Check sheet for the modelled part. Datum: model origin and axes. Units: mm. A direction names the side the tool comes from. Give positions to 0.01 mm unless a question says otherwise; leave off trailing zeros. Loops run counter-clockwise (first coordinate to the right, second up) from the corner with the lowest first, then second, coordinate; pieces in that order, holes last. Notation, with made-up numbers: M 2.25,27.5 L 43.25,27.5 A35 ccw 43.25,61.5 Z; hole C 39.5,-6.75 d3. An arc over 180 degrees is marked long. One line per question, with ' | ' between items. Start each with the question number.
Autodesk Inventor part; units mm, degrees
ref_plane "YZ Plane" through (0, 0, 0) normal (1, 0, 0) x (0, 1, 0)
ref_plane "XZ Plane" through (0, 0, 0) normal (0, 1, 0) x (-1, 0, 0)
ref_plane "XY Plane" through (0, 0, 0) normal (0, 0, 1) x (1, 0, 0)
sketch "Boceto2" plane through (0, 0, 0) normal (0, 1, 0) x (-1, 0, 0)
  line L0 (7.5, 100) -> (-7.5, 100)
  line L1 (-7.5, 100) -> (-7.5, -100)
  line L2 (-7.5, -100) -> (7.5, -100)
  line L3 (7.5, -100) -> (7.5, 100)
  line L4 (7.5, 100) -> (-7.5, -100) construction
  line L5 (-7.5, 100) -> (7.5, -100) construction
  point P0 (0, 0)
  dimension "d7" = 15
  dimension "d8" = 200
extrude "Extrusión1" add sketch "Boceto2" along normal blind 10
sketch "Boceto3" plane through (0, 10, 0) normal (0, 1, 0) x (1, 0, 0)
  circle A0 centre (3.25, 58.25) radius 1.75
  line L0 (5, 50) -> (-5, 50)
  line L1 (-5, 50) -> (-5, 60)
  line L2 (-5, 60) -> (5, 60)
  line L3 (5, 60) -> (5, 50)
  line L4 (5, 50) -> (-5, 60) construction
  line L5 (-5, 50) -> (5, 60) construction
  circle A1 centre (-3.25, 51.75) radius 1.75
  line L6 (7.5, 100) -> (-7.5, 100)
  line L7 (-7.5, 0) -> (3.408, 0)
  line L8 (5, -60) -> (5, -50)
  line L9 (-5, -60) -> (5, -60)
  line L10 (5, -50) -> (-5, -50)
  line L11 (-5, -50) -> (-5, -60)
  line L12 (-5, -50) -> (5, -60) construction
  circle A2 centre (-3.25, -51.75) radius 1.75
  line L13 (5, -50) -> (-5, -60) construction
  circle A3 centre (3.25, -58.25) radius 1.75
  line L14 (-7.5, -100) -> (7.5, -100)
  point P0 (0, 0)
  point P1 (-5, 55)
  point P2 (0, 100)
  point P3 (-5, -55)
  dimension "d11" = 3.5
  dimension "d12" = 1.75
  dimension "d13" = 1.75
  dimension "d14" = 1.75
  dimension "d15" = 1.75
  dimension "d16" = 10
  dimension "d17" = 10
  dimension "d19" = 40
  dimension "d81" = 40
hole "Agujero1" at (3.25, 10, 58.25) at (-3.25, 10, 51.75) at (3.25, 10, -58.25) at (-3.25, 10, -51.75) direction (0, -1, 0) diameter 3.5 end through all
sketch "Boceto4" plane through (0, 10, 0) normal (0, 1, 0) x (1, 0, 0)
  line L0 (-7.5, 100) -> (-7.5, -100)
  line L1 (-7.5, -100) -> (7.5, -100)
  line L2 (7.5, -100) -> (7.5, -80)
  line L3 (7.5, -80) -> (-7.5, -80)
  line L4 (-7.5, -80) -> (-7.5, -100)
  line L5 (-7.5, 0) -> (1.0116, 0)
  line L6 (-7.5, -100) -> (-7.5, 100)
  line L7 (-7.5, 100) -> (7.5, 100)
  line L8 (7.5, 100) -> (7.5, 80)
  line L9 (7.5, 80) -> (-7.5, 80)
  line L10 (-7.5, 80) -> (-7.5, 100)
  point P0 (0, 0)
  point P1 (-7.5, -80)
  point P2 (-7.5, 80)
  dimension "d27" = 15
  dimension "d28" = 20
extrude "Extrusión2" add sketch "Boceto4" along normal blind 80
sketch "Boceto5" plane through (0, 90, 0) normal (0, 1, 0) x (1, 0, 0)
  line L0 (-7.5, -100) -> (7.5, -100)
  line L1 (-7.5, -100) -> (49.5, -100)
  line L2 (49.5, -100) -> (49.5, 100)
  line L3 (49.5, 100) -> (-7.5, 100)
  line L4 (-7.5, 100) -> (-7.5, -100)
  line L5 (49.5, -100) -> (-150.5, -100)
  line L6 (-150.5, -100) -> (-150.5, 100)
  line L7 (-150.5, 100) -> (49.5, 100)
  line L8 (49.5, 100) -> (49.5, -100)
  point P0 (0, 0)
  point P1 (-7.5, 100)
  dimension "d31" = 57
  dimension "d32" = 200
  dimension "d75" = 200
extrude "Extrusión3" add sketch "Boceto5" along normal blind 110
sketch "Boceto6" plane through (0, 200, 0) normal (0, 1, 0) x (1, 0, 0)
  line L0 (49.5, 100) -> (7.5, 100)
  line L1 (49.5, 100) -> (29.5, 100)
  line L2 (29.5, 100) -> (29.5, 80)
  line L3 (7.5, -100) -> (49.5, -100)
  line L4 (28.5, -100) -> (28.5, -80)
  line L5 (-150.5, 100) -> (-150.5, -100)
  line L6 (29.5, 80) -> (-150.5, 80)
  line L7 (-150.5, 80) -> (-150.5, -80)
  line L8 (-150.5, -80) -> (29.5, -80)
  line L9 (29.5, -80) -> (29.5, 80)
  line L10 (-150.5, -100) -> (49.5, -100)
  point P0 (7.5, 80)
  point P1 (-50.5, -100)
  dimension "d36" = 20
  dimension "d37" = 20
  dimension "d38" = 20
  dimension "d77" = 20
extrude "Extrusión4" cut sketch "Boceto6" against normal blind 90 contours L8 L5 L6 L9
sketch "Boceto7" plane through (-150.5, 90, -100) normal (-1, 0, 0) x (0, 0, 1)
  line L0 (0, 110) -> (20, 110)
  line L1 (20, 110) -> (10, 110)
  line L2 (10, 110) -> (10, 20)
  line L3 (10, 20) -> (20, 20)
  line L4 (20, 20) -> (20, 110)
  line L5 (180, 110) -> (180, 20)
  line L6 (180, 110) -> (190, 110)
  line L7 (190, 110) -> (190, 20)
  line L8 (190, 20) -> (180, 20)
  line L9 (180, 20) -> (180, 110)
  line L10 (200, 0) -> (200, 110)
  line L11 (0, 0) -> (0, 110)
  line L12 (0, 110) -> (10, 110)
  line L13 (10, 110) -> (10, 20)
  line L14 (10, 20) -> (0, 20)
  line L15 (0, 20) -> (0, 110)
  line L16 (200, 110) -> (0, 110)
  line L17 (200, 110) -> (190, 110)
  line L18 (190, 110) -> (190, 20)
  line L19 (190, 20) -> (200, 20)
  line L20 (200, 20) -> (200, 110)
  point P0 (100, -90)
  dimension "d63" = 10
  dimension "d65" = 10
  dimension "d76" = 10
extrude "Extrusión5" cut sketch "Boceto7" against normal blind 30 contours L6 L7 L8 L5 | L0 L4 L3 L2
sketch "Boceto8" plane through (-7.5, 0, 100) normal (0, 0, 1) x (1, 0, 0)
  line L0 (-113, 110) -> (-113, 200)
  line L1 (-113, 200) -> (-113, 110)
  circle A0 centre (-124.75, 183.25) radius 1.75
  line L2 (-123, 175) -> (-133, 175)
  line L3 (-133, 175) -> (-133, 185)
  line L4 (-133, 185) -> (-123, 185)
  line L5 (-123, 185) -> (-123, 175)
  line L6 (-123, 175) -> (-133, 185) construction
  line L7 (-133, 175) -> (-123, 185) construction
  circle A1 centre (-131.25, 176.75) radius 1.75
  line L8 (-143, 200) -> (57, 200)
  line L9 (-143, 90) -> (-143, 200)
  line L10 (-113, 155) -> (-128, 155)
  line L11 (-123, 125) -> (-123, 135)
  line L12 (-133, 125) -> (-123, 125)
  line L13 (-123, 135) -> (-133, 125) construction
  line L14 (-123, 135) -> (-133, 135)
  line L15 (-133, 135) -> (-123, 125) construction
  circle A2 centre (-131.25, 133.25) radius 1.75
  line L16 (-133, 135) -> (-133, 125)
  circle A3 centre (-124.75, 126.75) radius 1.75
  line L17 (-143, 110) -> (-113, 110)
  point P0 (7.5, 0)
  point P1 (-133, 180)
  point P2 (-123, 180)
  point P3 (-133, 130)
  point P4 (-123, 130)
  dimension "d45" = 3.5
  dimension "d46" = 1.75
  dimension "d47" = 1.75
  dimension "d48" = 1.75
  dimension "d49" = 1.75
  dimension "d50" = 10
  dimension "d51" = 10
  dimension "d52" = 15
  dimension "d53" = 10
  dimension "d54" = 10
  dimension "d55" = 15
hole "Agujero2" at (-132.25, 183.25, 100) at (-138.75, 176.75, 100) at (-138.75, 133.25, 100) at (-132.25, 126.75, 100) direction (0, 0, -1) diameter 3.5 end through all
ref_plane "Plano de trabajo1" through (-150.5, 90, 100) normal (0, -1, 0) x (1, 0, 0)
split "Dividir1" plane through (-150.5, 90, 100) removes the side toward (0, -1, 0)
ref_plane "Plano de trabajo2" through (49.5, 90, 0) normal (0, 0, -1) x (-1, 0, 0)
ref_plane "Plano de trabajo3" through (-50.5, 90, 100) normal (1, 0, 0) x (0, 0, -1)
ref_plane "Plano de trabajo4" through (0, 145, 0) normal (0, 1, 0) x (1, 0, 0)
sketch "Boceto9" plane through (-150.5, 90, 100) normal (0, 0, 1) x (1, 0, 0)
  line L0 (85.0357, 30) -> (115.0357, 30)
  circle A0 centre (110.0357, 25) radius 1.75
  line L1 (90.0357, 25) -> (110.0357, 25)
  line L2 (115.0357, 30) -> (115.0357, 20)
  circle A1 centre (90.0357, 25) radius 1.75
  line L3 (85.0357, 20) -> (115.0357, 30) construction
  line L4 (85.0357, 30) -> (115.0357, 20) construction
  line L5 (85.0357, 20) -> (85.0357, 30)
  line L6 (115.0357, 20) -> (85.0357, 20)
  line L7 (200, 0) -> (200, 110)
  line L8 (200, 55) -> (88.2857, 55)
  circle A2 centre (90.0357, 85) radius 1.75
  line L9 (85.0357, 80) -> (115.0357, 80)
  line L10 (85.0357, 80) -> (115.0357, 90) construction
  line L11 (85.0357, 90) -> (85.0357, 80)
  line L12 (115.0357, 90) -> (85.0357, 90)
  line L13 (85.0357, 90) -> (115.0357, 80) construction
  circle A3 centre (110.0357, 85) radius 1.75
  line L14 (90.0357, 85) -> (110.0357, 85)
  line L15 (115.0357, 80) -> (115.0357, 90)
  line L16 (100.0357, 55) -> (185.099, 55) construction
  line L17 (160, 70) -> (160, 40)
  circle A4 centre (165, 45) radius 1.75
  line L18 (170, 40) -> (170, 70)
  line L19 (170, 70) -> (160, 40) construction
  line L20 (160, 40) -> (170, 40)
  line L21 (160, 70) -> (170, 40) construction
  circle A5 centre (165, 65) radius 1.75
  line L22 (165, 65) -> (165, 45)
  line L23 (170, 70) -> (160, 70)
  circle A6 centre (55, 65) radius 1.75
  line L24 (60, 70) -> (60, 40)
  line L25 (60, 40) -> (50, 40)
  circle A7 centre (55, 45) radius 1.75
  line L26 (55, 65) -> (55, 45)
  line L27 (60, 70) -> (50, 40) construction
  line L28 (50, 40) -> (50, 70)
  line L29 (50, 70) -> (60, 40) construction
  line L30 (50, 70) -> (60, 70)
  line L31 (30, 110) -> (30, 20)
  point P0 (150.5, -90)
  point P1 (100.0357, 34.7141)
  point P2 (100.0357, 34.7141)
  point P3 (85.0357, 36.6749)
  point P4 (115.0357, 25)
  point P5 (115.0357, 85)
  point P6 (189.1833, 40)
  point P7 (165, 70)
  point P8 (70.0357, 40)
  point P9 (55, 70)
  dimension "d89" = 10
  dimension "d90" = 30
  dimension "d91" = 5
  dimension "d92" = 5
  dimension "d93" = 5
  dimension "d94" = 5
  dimension "d95" = 30
  dimension "d96" = 5
  dimension "d97" = 5
  dimension "d98" = 3.5
  dimension "d99" = 5
  dimension "d100" = 5
  dimension "d101" = 5
  dimension "d102" = 5
  dimension "d103" = 5
  dimension "d104" = 20
hole "Agujero3" at (-60.4643, 175, 100) at (-40.4643, 175, 100) at (14.5, 155, 100) at (-95.5, 155, 100) at (-95.5, 135, 100) at (-60.4643, 115, 100) at (-40.4643, 115, 100) at (14.5, 135, 100) direction (0, 0, -1) diameter 3.5 end through all
sketch "Boceto10" plane through (49.5, 90, 100) normal (1, 0, 0) x (0, 0, -1)
  line L0 (85.0357, 30) -> (115.0357, 30)
  circle A0 centre (110.0357, 25) radius 1.75
  line L1 (90.0357, 25) -> (110.0357, 25)
  line L2 (115.0357, 30) -> (115.0357, 20)
  circle A1 centre (90.0357, 25) radius 1.75
  line L3 (85.0357, 30) -> (115.0357, 20) construction
  line L4 (85.0357, 20) -> (85.0357, 30)
  line L5 (115.0357, 20) -> (85.0357, 20)
  line L6 (85.0357, 20) -> (115.0357, 30) construction
  line L7 (160, 70) -> (160, 40)
  circle A2 centre (165, 45) radius 1.75
  line L8 (160, 40) -> (170, 40)
  line L9 (165, 65) -> (165, 45)
  circle A3 centre (165, 65) radius 1.75
  line L10 (170, 70) -> (160, 40) construction
  line L11 (170, 70) -> (160, 70)
  line L12 (160, 70) -> (170, 40) construction
  line L13 (170, 40) -> (170, 70)
  line L14 (40, 70) -> (40, 40)
  line L15 (35, 65) -> (35, 45)
  circle A4 centre (35, 65) radius 1.75
  line L16 (40, 40) -> (30, 40)
  line L17 (40, 70) -> (30, 40) construction
  line L18 (30, 70) -> (40, 40) construction
  line L19 (30, 70) -> (40, 70)
  line L20 (30, 40) -> (30, 70)
  circle A5 centre (35, 45) radius 1.75
  circle A6 centre (90.0357, 85) radius 1.75
  line L21 (85.0357, 80) -> (115.0357, 80)
  line L22 (115.0357, 80) -> (115.0357, 90)
  circle A7 centre (110.0357, 85) radius 1.75
  line L23 (90.0357, 85) -> (110.0357, 85)
  line L24 (85.0357, 80) -> (115.0357, 90) construction
  line L25 (85.0357, 90) -> (85.0357, 80)
  line L26 (115.0357, 90) -> (85.0357, 90)
  line L27 (85.0357, 90) -> (115.0357, 80) construction
  line L28 (0, 0) -> (0, 110)
  line L29 (200, 0) -> (200, 110)
  point P0 (100, -90)
  point P1 (100.0357, 34.7141)
  point P2 (100.0357, 34.7141)
  point P3 (85.0357, 36.6749)
  point P4 (115.0357, 25)
  point P5 (88.2857, 55)
  point P6 (189.1833, 40)
  point P7 (165, 70)
  point P8 (70.0357, 40)
  point P9 (35, 70)
  point P10 (115.0357, 85)
  point P11 (100.0357, 55)
  dimension "d112" = 10
  dimension "d113" = 30
  dimension "d114" = 5
  dimension "d115" = 5
  dimension "d116" = 5
  dimension "d117" = 5
  dimension "d118" = 5
  dimension "d119" = 5
  dimension "d120" = 3.5
  dimension "d121" = 5
  dimension "d122" = 5
  dimension "d123" = 5
  dimension "d124" = 5
  dimension "d125" = 5
  dimension "d126" = 30
  dimension "d127" = 30
hole "Agujero4" at (49.5, 175, 9.9643) at (49.5, 175, -10.0357) at (49.5, 155, 65) at (49.5, 135, 65) at (49.5, 115, 9.9643) at (49.5, 115, -10.0357) at (49.5, 135, -65) at (49.5, 155, -65) direction (-1, 0, 0) diameter 3.5 end through all
properties part number "container_front_head"
Q1. Access from +Z, -Z, +X, -X, +Y, -Y to the whole of each face (thin tool, end or side, straight path). Record for faces 1 (the flat face through (-120.5, 156, 85)), 2 (the flat face through (31, 200, 7)).
Q2. Cross-section at A-A (x = -107). Record the cut outline in (y, z), and give its area (3 significant figures).
Q3. Cross-section at B-B (y = 142). Record the cut outline in (x, z), and give its area (3 significant figures).
Q4. Material ranges on probe 1 along X at (y, z) = (175, 87.25); probe 2 along Y at (x, z) = (-132, -93); probe 3 along Z at (x, y) = (43.25, 115), recorded low to high. Write a range as from..to.
Q5. Depth check by flat-ended pin: P1, Ø4, axis at x = 14.5, y = 135, coming from the +Z side; P2, Ø10, axis at x = -103, z = -66, coming from the +Y side; P3, Ø3, axis at y = 140, z = -85, coming from the -X side; P4, Ø3, axis at y = 115, z = 9.96, coming from the -X side. Enter the tip coordinate at first touch or a pass-through.
Q6. Cross-section at C-C (z = -37). Record the cut outline in (x, y), and give its area (3 significant figures).
Q7. Draft check along Z on faces 3 (the flat face through (-49, 144, -100)), 4 (the flat face through (-44, 156, -80)), 5 (the flat face through (-52, 144, 100)), 6 (the flat face through (49.5, 144, 1)). Enter one of: released by +Z, released by -Z, zero draft, split by the parting line, or undercut.
Solved:
1) face 1: -X, +Y | face 2: +Z, -Z, +X, -X, +Y
2) outline: M 90,-100 L 200,-100 L 200,-80 L 110,-80 L 110,80 L 200,80 L 200,100 L 90,100 Z | area: 7,600 mm²
3) outline: M -150.5,-100 L 49.5,-100 L 49.5,100 L -150.5,100 L -150.5,90 L -120.5,90 L -120.5,80 L 29.5,80 L 29.5,-80 L -120.5,-80 L -120.5,-90 L -150.5,-90 Z | area: 10,600 mm²
4) probe 1: x = -120.5..-62.21, -58.71..-42.21, -38.71..49.5 | probe 2: y = 90..125.02, 128.48..181.52, 184.98..200 | probe 3: z = -100..-11.79, -8.29..8.21, 11.71..100
5) P1: stops at z = 100 | P2: stops at y = 110 | P3: stops at x = -120.5 | P4: passes through
6) outline: M -150.5,90 L 49.5,90 L 49.5,200 L 29.5,200 L 29.5,110 L -150.5,110 Z | area: 5,800 mm²
7) face 3: released by -Z | face 4: undercut | face 5: released by +Z | face 6: zero draft
